Design review of the part shown in the three views and the two pictorial views. Dimensions are in mm from the part's minimum x, y and z. Round coordinates to 2 decimals unless told otherwise and drop trailing zeros. Loops run counter-clockwise (first coordinate to the right, second up) from the corner with the lowest first, then second, coordinate; pieces in that order, holes last.
1) Take a section at C-C (y = 0.15). State the section outline as (x, z) points.
2) Take a section at B-B (x = 57). State the section outline as (y, z) points, then the cut area to 3 significant figures.
3) Insertion check: pin 1 (10 mm diameter, centred on x = 23.5, z = 7.5, fed in from -Y). The pin has a flat end and moves straight along its axis. Give the tip position at first contact, or say it passes through.
4) Take a section at D-D (z = 34.5). State the section outline as (x, y) points, then the cut area to 3 significant figures.
5) Wall thickness on L1, parallel to X at y = 0.55, z = 54.8; L2, parallel to X at y = 0.65, z = 19; L3, parallel to Z at x = 38, y = 0.05: over which ranges is each line inside the solid? List them lowest first.
6) Take a section at A-A (z = 54.8). State the section outline as (x, y) points.
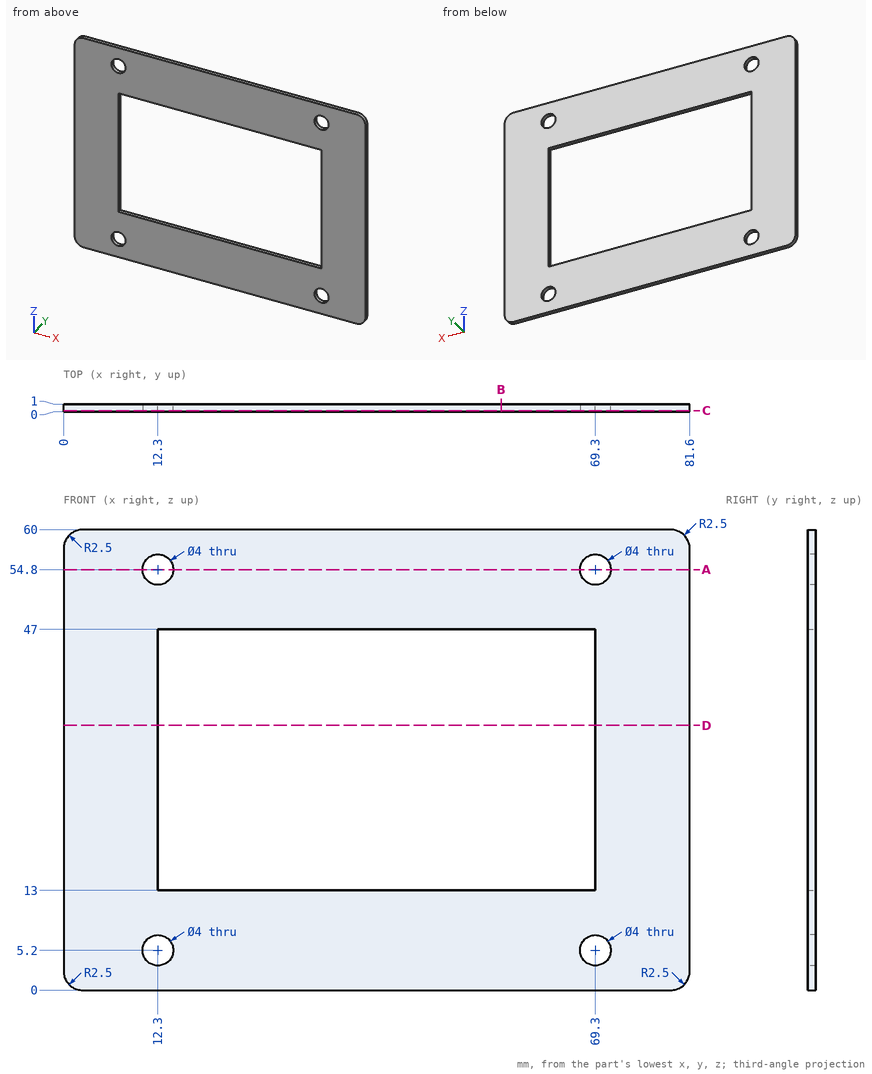
Response:
1. outline: (0, 2.5) arc R2.5 ccw to (2.5, 0) - (79.1, 0) arc R2.5 ccw to (81.6, 2.5) - (81.6, 57.5) arc R2.5 ccw to (79.1, 60) - (2.5, 60) arc R2.5 ccw to (0, 57.5) - close; hole circle Ø4 at (12.3, 5.2); hole circle Ø4 at (12.3, 54.8); hole (12.3, 13) - (69.3, 13) - (69.3, 47) - (12.3, 47) - close; hole circle Ø4 at (69.3, 5.2); hole circle Ø4 at (69.3, 54.8)
2. outline: (0, 0) - (1, 0) - (1, 13) - (0, 13) - close; (0, 47) - (1, 47) - (1, 60) - (0, 60) - close
2. area: 26.0 mm2
3. pin 1: stops at y = 0
4. outline: (0, 0) - (12.3, 0) - (12.3, 1) - (0, 1) - close; (69.3, 0) - (81.6, 0) - (81.6, 1) - (69.3, 1) - close
4. area: 24.6 mm2
5. L1: x = 0 to 10.3, 14.3 to 67.3, 71.3 to 81.6
5. L2: x = 0 to 12.3, 69.3 to 81.6
5. L3: z = 0 to 13, 47 to 60
6. outline: (0, 0) - (10.3, 0) - (10.3, 1) - (0, 1) - close; (14.3, 0) - (67.3, 0) - (67.3, 1) - (14.3, 1) - close; (71.3, 0) - (81.6, 0) - (81.6, 1) - (71.3, 1) - close
